```python
from build123d import *

# Parameters (mm, degrees)
SKETCH_1_W          = 7
SKETCH_1_H          = 4.3
EXTRUDE_1_DEPTH     = 2.65
EXTRUDE_2_DEPTH     = 1.2
SKETCH_3_W          = 4.5
SKETCH_3_H          = 4.3
EXTRUDE_2_2_DEPTH   = 0.08
SKETCH_4_W          = 0.3
SKETCH_4_H          = 4.3
EXTRUDE_3_DEPTH     = 0.02
MOVE_START          = -2.15
MOVE_BODY_1_DEPTH   = 4.3
MOVE_BODY_1_2_DEPTH = 0.95
MOVE_START_2        = 1.2
MOVE_BODY_1_3_DEPTH = 0.95
MOVE_BODY_1_4_DEPTH = 4.3
MOVE_START_3        = -1.2
MOVE_BODY_1_5_DEPTH = 2.4


# Read off the part's stored shape, not the designer's step: Тело-Переместить/Копировать1
with BuildPart() as part:
    # Эскиз1 → Бобышка-Вытянуть1 (new body)
    with BuildSketch(Plane.XY):
        Rectangle(SKETCH_1_W, SKETCH_1_H)
    extrude(amount=EXTRUDE_1_DEPTH)

    # Эскиз2 → Extrude 2 (add, symmetric)
    with BuildSketch(Plane(origin=(0, 0, 0), x_dir=(1, 0, 0), z_dir=(0, 1, 0))):
        with BuildLine():
            Line((-3.5, -1.275), (-3.55, -1.275))
            Line((-3.55, -1.275), (-3.55, 0.05))
            Line((-3.55, 0.05), (-2.35, 0.05))
            Line((-2.35, 0.05), (-2.35, 0.15))
            Line((-2.35, 0.15), (-3.568137941, 0.15))
            ThreePointArc((-3.568137941, 0.15), (-3.626023158, 0.126023158), (-3.65, 0.068137941))
            Line((-3.65, 0.068137941), (-3.65, -1.293137941))
            ThreePointArc((-3.65, -1.293137941), (-3.626023158, -1.351023158), (-3.568137941, -1.375))
            Line((-3.568137941, -1.375), (-3.5, -1.375))
            Line((-3.5, -1.375), (-3.5, -1.275))
        make_face()
    extrude_2 = extrude(amount=EXTRUDE_2_DEPTH, both=True)

    # Эскиз3 → Extrude 2 2 (add)
    with BuildSketch(Plane(origin=(0, 0, 0), x_dir=(-1, 0, 0), z_dir=(0, 0, -1))):
        Rectangle(SKETCH_3_W, SKETCH_3_H)
    extrude(amount=EXTRUDE_2_2_DEPTH)

    # Зеркальное отражение1: Extrude 2 across plane
    add(extrude_2.mirror(Plane(origin=(0, 0, 0), x_dir=(0, 0, 1), z_dir=(1, 0, 0))))

    # Эскиз4 → Бобышка-Вытянуть3 (add)
    with BuildSketch(Plane.XY.offset(2.65)):
        with Locations((-3.25, 0)):
            Rectangle(SKETCH_4_W, SKETCH_4_H)
    extrude(amount=EXTRUDE_3_DEPTH)

    # Move Body 1 outline → Move Body 1 (cut)
    with BuildSketch(Plane(origin=(0, 0, 0), x_dir=(1, 0, 0), z_dir=(0, 1, 0)).offset(MOVE_START)):
        with BuildLine():
            Line((-3.1, -2.65), (-0.525, -2.65))
            Line((-0.525, -2.65), (-0.525, -1.525))
            Line((-0.525, -1.525), (-0.593137941, -1.525))
            ThreePointArc((-0.593137941, -1.525), (-0.651023158, -1.501023158), (-0.675, -1.443137941))
            Line((-0.675, -1.443137941), (-0.675, -0.081862059))
            ThreePointArc((-0.675, -0.081862059), (-0.651023158, -0.023976842), (-0.593137941, 0))
            Line((-0.593137941, 0), (0.625, 0))
            Line((0.625, 0), (0.625, -0.1))
            Line((0.625, -0.1), (-0.575, -0.1))
            Line((-0.575, -0.1), (-0.575, -1.425))
            Line((-0.575, -1.425), (-0.525, -1.425))
            Line((-0.525, -1.425), (-0.525, -0.15))
            Line((-0.525, -0.15), (0.725, -0.15))
            Line((0.725, -0.15), (0.725, -0.07))
            Line((0.725, -0.07), (3.5, -0.07))
            Line((3.5, -0.07), (3.5, 0))
            Line((3.5, 0), (2.25, 0))
            Line((2.25, 0), (2.25, 0.08))
            Line((2.25, 0.08), (-2.25, 0.08))
            Line((-2.25, 0.08), (-2.25, 0))
            Line((-2.25, 0), (-3.5, 0))
            Line((-3.5, 0), (-3.5, -1.275))
            Line((-3.5, -1.275), (-3.55, -1.275))
            Line((-3.55, -1.275), (-3.55, 0.05))
            Line((-3.55, 0.05), (-2.35, 0.05))
            Line((-2.35, 0.05), (-2.35, 0.15))
            Line((-2.35, 0.15), (-3.568137941, 0.15))
            ThreePointArc((-3.568137941, 0.15), (-3.626023158, 0.126023158), (-3.65, 0.068137941))
            Line((-3.65, 0.068137941), (-3.65, -1.293137941))
            ThreePointArc((-3.65, -1.293137941), (-3.626023158, -1.351023158), (-3.568137941, -1.375))
            Line((-3.568137941, -1.375), (-3.5, -1.375))
            Line((-3.5, -1.375), (-3.5, -2.65))
            Line((-3.5, -2.65), (-3.4, -2.65))
            Line((-3.4, -2.65), (-3.4, -2.67))
            Line((-3.4, -2.67), (-3.1, -2.67))
            Line((-3.1, -2.67), (-3.1, -2.65))
        make_face()
        with BuildLine():
            Line((3.55, 0.05), (3.55, -0.07))
            Line((3.55, -0.07), (3.65, -0.07))
            Line((3.65, -0.07), (3.65, 0.068137941))
            ThreePointArc((3.65, 0.068137941), (3.626023158, 0.126023158), (3.568137941, 0.15))
            Line((3.568137941, 0.15), (2.35, 0.15))
            Line((2.35, 0.15), (2.35, 0.05))
            Line((2.35, 0.05), (3.55, 0.05))
        make_face()
    extrude(amount=MOVE_BODY_1_DEPTH, mode=Mode.SUBTRACT)

    # Move Body 1 2 outline → Move Body 1 2 (cut)
    with BuildSketch(Plane(origin=(0, 0, 0), x_dir=(1, 0, 0), z_dir=(0, 1, 0)).offset(MOVE_START)):
        with BuildLine():
            Line((-0.593137941, -1.525), (-0.525, -1.525))
            Line((-0.525, -1.525), (-0.525, -1.425))
            Line((-0.525, -1.425), (-0.575, -1.425))
            Line((-0.575, -1.425), (-0.575, -0.1))
            Line((-0.575, -0.1), (0.625, -0.1))
            Line((0.625, -0.1), (0.625, 0))
            Line((0.625, 0), (-0.593137941, 0))
            ThreePointArc((-0.593137941, 0), (-0.651023158, -0.023976842), (-0.675, -0.081862059))
            Line((-0.675, -0.081862059), (-0.675, -1.443137941))
            ThreePointArc((-0.675, -1.443137941), (-0.651023158, -1.501023158), (-0.593137941, -1.525))
        make_face()
    extrude(amount=MOVE_BODY_1_2_DEPTH, mode=Mode.SUBTRACT)

    # Move Body 1 3 outline → Move Body 1 3 (cut)
    with BuildSketch(Plane(origin=(0, 0, 0), x_dir=(1, 0, 0), z_dir=(0, 1, 0)).offset(MOVE_START_2)):
        with BuildLine():
            Line((-0.593137941, -1.525), (-0.525, -1.525))
            Line((-0.525, -1.525), (-0.525, -1.425))
            Line((-0.525, -1.425), (-0.575, -1.425))
            Line((-0.575, -1.425), (-0.575, -0.1))
            Line((-0.575, -0.1), (0.625, -0.1))
            Line((0.625, -0.1), (0.625, 0))
            Line((0.625, 0), (-0.593137941, 0))
            ThreePointArc((-0.593137941, 0), (-0.651023158, -0.023976842), (-0.675, -0.081862059))
            Line((-0.675, -0.081862059), (-0.675, -1.443137941))
            ThreePointArc((-0.675, -1.443137941), (-0.651023158, -1.501023158), (-0.593137941, -1.525))
        make_face()
    extrude(amount=MOVE_BODY_1_3_DEPTH, mode=Mode.SUBTRACT)

    # Move Body 1 4 outline → Move Body 1 4 (add)
    with BuildSketch(Plane(origin=(0, 0, 0), x_dir=(1, 0, 0), z_dir=(0, 1, 0)).offset(MOVE_START)):
        Polygon((-0.525, -2.8), (-0.425, -2.8), (-0.425, -2.82), (-0.125, -2.82), (-0.125, -2.8), (6.475, -2.8), (6.475, -0.15), (5.225, -0.15), (5.225, -0.07), (3.5, -0.07), (3.5, -2.65), (-0.525, -2.65), align=None)
    extrude(amount=MOVE_BODY_1_4_DEPTH)

    # Move Body 1 5 outline → Move Body 1 5 (add)
    with BuildSketch(Plane(origin=(0, 0, 0), x_dir=(1, 0, 0), z_dir=(0, 1, 0)).offset(MOVE_START_3)):
        with BuildLine():
            Line((6.475, -1.425), (6.475, -1.525))
            Line((6.475, -1.525), (6.543137941, -1.525))
            ThreePointArc((6.543137941, -1.525), (6.601023158, -1.501023158), (6.625, -1.443137941))
            Line((6.625, -1.443137941), (6.625, -0.081862059))
            ThreePointArc((6.625, -0.081862059), (6.601023158, -0.023976842), (6.543137941, 0))
            Line((6.543137941, 0), (5.325, 0))
            Line((5.325, 0), (5.325, -0.1))
            Line((5.325, -0.1), (6.525, -0.1))
            Line((6.525, -0.1), (6.525, -1.425))
            Line((6.525, -1.425), (6.475, -1.425))
        make_face()
    extrude(amount=MOVE_BODY_1_5_DEPTH)


solid = part.part
```
Can you work these out from the model? Positions are in its coordinate system, mm. Give positions to 0.01 mm unless a question says otherwise; leave off trailing zeros. Order: outer loops, then holes, each group sorted by start corner. A loop starts at its lowest first (then second) coordinate and runs counter-clockwise, first axis right, second up. Notation, with made-up numbers: (89, 71) - (122, 71) arc R23 ccw to (122, 86) - close; hole circle Ø8 at (2, 48.25). An arc over 180 degrees is marked (long way). Use a Markdown table: item, result. Add a question column.
Q1. If we section it at A-A on z = 1.05: Write out the boundary of the cut face in (x, y) (3 decimals).
Q2. Please list where these lines run through material, in increasing order: line 1 along Z through (x, y) = (3, 0.8); line 2 along X through (y, z) = (1.8, 1.7) (3 decimals); line 3 along Z through (x, y) = (6, -1.45).
Q3. If we section it at D-D on x = 4: Write out the boundary of the cut face in (y, z), plus the area to 3 significant figures.
Q4. If we section it at B-B on x = 5.75: Write out the boundary of the cut face in (y, z), plus the area to 3 significant figures.
Q5. I'm going to push a flat-ended pin straight in: pin 1 (1.3 mm diameter, centred on x = 6, y = 0, fed in from +Z). Where does the tip first touch, or does it pass through?
Q6. If we mould it in two halves opening along Z, with no side actions, what happens to faces 1 (the flat face through (-0.525, 0, 2)), 2 (the flat face through (3, 0, 2.8)), 3 (the flat face through (3, 2.15, 1))? For each: released by +Z, released by -Z, zero draft, split by the parting line, or undercut.
Answers follow:
| question | item | result |
|---|---|---|
| 1 | outline | (-0.675, -1.2) - (-0.575, -1.2) - (-0.575, 1.2) - (-0.675, 1.2) - close; (-0.525, -2.15) - (6.475, -2.15) - (6.475, 2.15) - (-0.525, 2.15) - close; (6.525, -1.2) - (6.625, -1.2) - (6.625, 1.2) - (6.525, 1.2) - close |
| 2 | line 1 | z = 0.07 to 2.8 |
| 2 | line 2 | x = -0.525 to 6.475 |
| 2 | line 3 | z = 0.15 to 2.8 |
| 3 | outline | (-2.15, 0.07) - (2.15, 0.07) - (2.15, 2.8) - (-2.15, 2.8) - close |
| 3 | area | 11.7 mm^2 |
| 4 | outline | (-2.15, 0.15) - (2.15, 0.15) - (2.15, 2.8) - (-2.15, 2.8) - close; (-1.2, 0) - (1.2, 0) - (1.2, 0.1) - (-1.2, 0.1) - close |
| 4 | area | 11.6 mm^2 |
| 5 | pin 1 | stops at z = 2.8 |
| 6 | face 1 | undercut |
| 6 | face 2 | released by +Z |
| 6 | face 3 | zero draft |
